Source: three-view drawing plus pictorial views. Frame: mm from the lowest corner of the part. Give positions to 0.01 mm unless a question says otherwise; leave off trailing zeros. Order: outer loops, then holes, each group sorted by start corner. A loop starts at its lowest first (then second) coordinate and runs counter-clockwise, first axis right, second up.
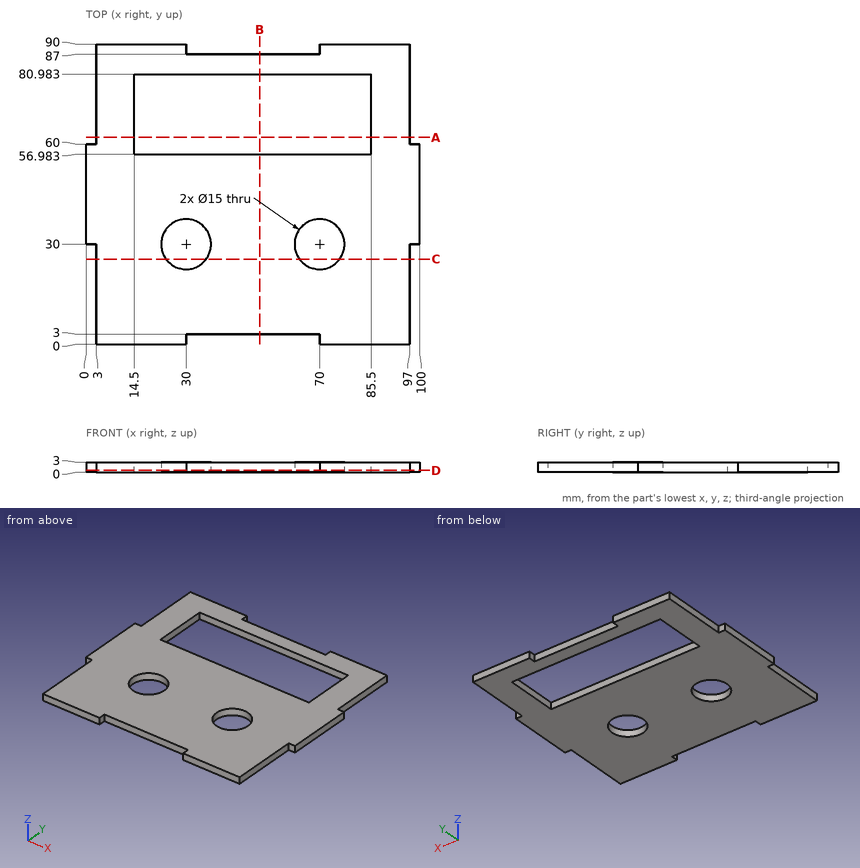
1) Ray query, L1, parallel to Y at x = 51, z = 1.15; L2, parallel to X at y = 63, z = 2.8; L3, parallel to Y at x = 76.5, z = 2.25 (1 decimal). Return the intervals inside material, ascending.
Checks:
L1: y = 3 to 56.98, 80.98 to 87
L2: x = 3 to 14.5, 85.5 to 97
L3: y = 0 to 26.3, 33.7 to 57, 81 to 90
2) Section query B-B on x = 52. Output: boundary loops of the cut face in (y, z), and give its area (3 significant figures).
Checks:
outline: (3, 0) - (56.98, 0) - (56.98, 3) - (3, 3) - close; (80.98, 0) - (87, 0) - (87, 3) - (80.98, 3) - close
area: 180 mm2
3) First-contact query: pin 1 Ø0.9 at (y, z) = (8, 1) entering from +X; pin 2 Ø1.5 at (x, z) = (49.5, 1.5) entering from -Y; pin 3 Ø1 at (x, z) = (63, 0.5) entering from +Y. Flat tips, straight axial feed; report the tip coordinate or a pass-through.
Checks:
pin 1: stops at x = 97
pin 2: stops at y = 3
pin 3: stops at y = 87
4) Section query C-C on y = 25.5. Output: boundary loops of the cut face in (x, z).
Checks:
outline: (3, 0) - (24, 0) - (24, 3) - (3, 3) - close; (36, 0) - (64, 0) - (64, 3) - (36, 3) - close; (76, 0) - (97, 0) - (97, 3) - (76, 3) - close
5) Section query A-A on y = 62. Output: boundary loops of the cut face in (x, z).
Checks:
outline: (3, 0) - (14.5, 0) - (14.5, 3) - (3, 3) - close; (85.5, 0) - (97, 0) - (97, 3) - (85.5, 3) - close
6) Section query D-D on z = 0.55. Output: boundary loops of the cut face in (x, y).
Checks:
outline: (0, 30) - (3, 30) - (3, 0) - (30, 0) - (30, 3) - (70, 3) - (70, 0) - (97, 0) - (97, 30) - (100, 30) - (100, 60) - (97, 60) - (97, 90) - (70, 90) - (70, 87) - (30, 87) - (30, 90) - (3, 90) - (3, 60) - (0, 60) - close; hole (14.5, 56.98) - (85.5, 56.98) - (85.5, 80.98) - (14.5, 80.98) - close; hole circle Ø15 at (30, 30); hole circle Ø15 at (70, 30)
